Could you check a few things on this model? Use its own coordinates, in mm. A direction names the side the tool comes from. Coordinates: 2 decimals unless noted, no trailing zeros. Write each loop counter-clockwise with the first axis right and the second up, starting at its lowest first coordinate (ties: lowest second). Pieces come first, ordered by that corner, then holes.
```python
from build123d import *

# Parameters (mm, degrees)
SKETCH2_W           = 107
SKETCH2_H           = 10
BOSS_EXTRUDE1_DEPTH = 48.42
BOSS_EXTRUDE2_DEPTH = 48.42
BOSS_EXTRUDE3_DEPTH = 2.54
BOSS_EXTRUDE4_DEPTH = 2.54
FILLET1_R           = 3


with BuildPart() as part:
    # Sketch2 → Boss-Extrude1 (new body)
    with BuildSketch(Plane.XY):
        with Locations((53.5, 5)):
            Rectangle(SKETCH2_W, SKETCH2_H)
    extrude(amount=BOSS_EXTRUDE1_DEPTH)

    # Sketch3 → Boss-Extrude2 (add)
    with BuildSketch(Plane.XY.offset(48.42)):
        Polygon((107, 10), (117, 10), (117, -10), (147, -10), (147, -20), (117, -20), (107, -20), align=None)
    extrude(amount=-BOSS_EXTRUDE2_DEPTH)

    # Sketch4 → Boss-Extrude3 (add)
    with BuildSketch(Plane.XY.offset(48.42)):
        Polygon((-2.54, 12.54), (119.54, 12.54), (119.54, -7.46), (149.54, -7.46), (149.54, -22.54), (104.46, -22.54), (104.46, -2.54), (-2.54, -2.54), align=None)
    extrude(amount=BOSS_EXTRUDE3_DEPTH)

    # Sketch5 → Boss-Extrude4 (add)
    with BuildSketch(Plane(origin=(0, 0, 0), x_dir=(-1, 0, 0), z_dir=(0, 0, -1))):
        Polygon((-119.54, 12.54), (-119.54, -7.46), (-149.54, -7.46), (-149.54, -22.54), (-104.46, -22.54), (-104.46, -2.54), (2.54, -2.54), (2.54, 12.54), align=None)
    extrude(amount=BOSS_EXTRUDE4_DEPTH)

    # Fillet1
    fillet1_edges = [part.edges().sort_by_distance(p)[0] for p in [
        (107, -20, 24.21),
        (117, 10, 24.21),
        (117, -10, 24.21),
        (147, -10, 24.21),
        (147, -20, 24.21),
        (-2.54, 12.54, 49.69),
        (-2.54, -2.54, 49.69),
        (104.46, -2.54, 49.69),
        (104.46, -22.54, 49.69),
        (149.54, -22.54, 49.69),
        (149.54, -7.46, 49.69),
        (119.54, -7.46, 49.69),
        (119.54, 12.54, 49.69),
        (149.54, -7.46, -1.27),
        (149.54, -22.54, -1.27),
        (104.46, -22.54, -1.27),
        (104.46, -2.54, -1.27),
        (-2.54, -2.54, -1.27),
        (-2.54, 12.54, -1.27),
        (119.54, 12.54, -1.27),
        (119.54, -7.46, -1.27),
        (0, 10, 24.21),
        (107, 0, 24.21),
    ]]
    fillet(fillet1_edges, radius=FILLET1_R)


solid = part.part
```
1. I want a section at A-A on z = 26.5. Please give me the cut outline in (x, y).
Verdict:
outline: (0, 0) - (104, 0) arc R3 cw to (107, -3) - (107, -17) arc R3 ccw to (110, -20) - (144, -20) arc R3 ccw to (147, -17) - (147, -13) arc R3 ccw to (144, -10) - (120, -10) arc R3 cw to (117, -7) - (117, 7) arc R3 ccw to (114, 10) - (3, 10) arc R3 ccw to (0, 7) - close
2. For pin 1 (24 mm diameter, centred on x = 63.5, z = 15, fed in from -Y); pin 2 (8 mm diameter, centred on x = 26, y = -9.5, fed in from +Z); pin 3 (3 mm diameter, centred on y = -15, z = 24.5, fed in from +X); pin 4 (3 mm diameter, centred on x = 47.5, z = 7.5, fed in from +Y), each with a flat end and sliding along its axis, tell me the tip position at first contact or that it passes through.
Verdict:
pin 1: stops at y = 0
pin 2: passes through
pin 3: stops at x = 147
pin 4: stops at y = 10
3. I want a section at B-B on x = 82. Please give me the cut outline in (y, z), plus the area to 3 significant figures.
Verdict:
outline: (-2.54, -2.54) - (12.54, -2.54) - (12.54, 0) - (10, 0) - (10, 48.42) - (12.54, 48.42) - (12.54, 50.96) - (-2.54, 50.96) - (-2.54, 48.42) - (0, 48.42) - (0, 0) - (-2.54, 0) - close
area: 561 mm2
4. If we mould it in two halves opening along Z, with no side actions, what happens to faces 1 (the face through (-1.68, -1.64, -1.29)), 2 (the face through (75, -1, -2.54)), 3 (the face through (116.14, 9.1, 23.87))? For each: pulls with the +Z half, pulls with the -Z half, needs draft (parallel to the pull), parting line crosses it, or undercut.
Verdict:
face 1: needs draft
face 2: pulls with the -Z half
face 3: undercut
5. Please list where these lines run through material, in increasing order: line 1 along Z through (x, y) = (118, 6); line 2 along Y through (x, z) = (133, 13); line 3 along Y through (x, z) = (11, 34).
Verdict:
line 1: z = -2.54 to 0, 48.42 to 50.96
line 2: y = -20 to -10
line 3: y = 0 to 10
6. I want a section at C-C on y = 5. Please give me the cut outline in (x, z).
Verdict:
outline: (-2.54, -2.54) - (119.54, -2.54) - (119.54, 0) - (117, 0) - (117, 48.42) - (119.54, 48.42) - (119.54, 50.96) - (-2.54, 50.96) - (-2.54, 48.42) - (0, 48.42) - (0, 0) - (-2.54, 0) - close
7. On a 3-axis mill with a long thin cutter (end or side, diameter ignored), from which of +Z, -Z, +X, -X, +Y, -Y can I reach the whole of each face in a straight line? I mean faces 4 (the face through (107.9, -19.14, 23.87)), 5 (the face through (117.86, -9.1, 23.87)), 6 (the face through (85, -2, 0)), 7 (the face through (58, 10, 25)), 8 (the face through (127, -20, 25)). Say none if no direction works.
Verdict:
face 4: -X, -Y
face 5: +X, +Y
face 6: none
face 7: +X, -X, +Y
face 8: +X, -X, -Y
